```python
from build123d import *

# Parameters (mm, degrees)
SKETCH1_R                = 7
SKETCH1_R_2              = 3.5
CYLINDER_DEPTH           = 22.85
SKETCH2_R                = 4
BORE_1_DEPTH             = 3.25
BORE_START               = -3.25
SKETCH3_R                = 4
BORE_2_DEPTH             = 3.25
ARM_DEPTH                = 17
SKETCH5_R                = 3.5
OUTER_HOLE_SURFACE_DEPTH = 6
SKETCH6_R                = 1.125
OUTER_HOLE_DEPTH         = 6
SIDE_FEATURES_DEPTH      = 22
RIB_START                = -11
SKETCH10_W               = 6.681980515
SKETCH10_H               = 4.897943925
RIB_DEPTH                = 9.5
SKETCH13_R               = 1.5
BOTTOM_HOLE_DEPTH        = 4


# Read off the part's stored shape, not the designer's step: Top Counter-sunk
with BuildPart() as part:
    # Sketch1 → Cylinder (new body)
    with BuildSketch(Plane.XY):
        with Locations(Location((0, 0, 0), (0, 0, 180))):
            Circle(SKETCH1_R)
        with Locations(Location((0, 0, 0), (0, 0, 180))):
            Circle(SKETCH1_R_2, mode=Mode.SUBTRACT)
    extrude(amount=CYLINDER_DEPTH)

    # Sketch2 → Bore 1 (cut)
    with BuildSketch(Plane.XY.offset(22.85)):
        Circle(SKETCH2_R)
    extrude(amount=-BORE_1_DEPTH, mode=Mode.SUBTRACT)

    # Sketch3 → Bore 2 (cut)
    with BuildSketch(Plane(origin=(0, 0, 0), x_dir=(-1, 0, 0), z_dir=(0, 0, -1)).offset(BORE_START)):
        with Locations(Location((0, 0, 0), (0, 0, 180))):
            Circle(SKETCH3_R)
    extrude(amount=BORE_2_DEPTH, mode=Mode.SUBTRACT)

    # Sketch4 → Arm (add)
    with BuildSketch(Plane.XY):
        with BuildLine():
            Line((0.734153157, 6.961394914), (30, 3.875))
            ThreePointArc((30, 3.875), (33.875, 0), (30, -3.875))
            Line((30, -3.875), (0.734153157, -6.961394914))
            ThreePointArc((0.734153157, -6.961394914), (7, 0), (0.734153157, 6.961394914))
        make_face()
    extrude(amount=ARM_DEPTH)

    # Sketch5 → Outer Hole surface (add)
    with BuildSketch(Plane(origin=(0, 0, 0), x_dir=(-1, 0, 0), z_dir=(0, 0, -1))):
        with Locations((-14, 6)):
            Circle(SKETCH5_R)
    extrude(amount=-OUTER_HOLE_SURFACE_DEPTH)

    # Sketch6 → Outer hole (cut)
    with BuildSketch(Plane(origin=(0, 0, 0), x_dir=(-1, 0, 0), z_dir=(0, 0, -1))):
        with Locations((-14, 6)):
            Circle(SKETCH6_R)
    extrude(amount=-OUTER_HOLE_DEPTH, mode=Mode.SUBTRACT)

    # Sketch8 → side Features (cut)
    with BuildSketch(Plane(origin=(0, 10, 0), x_dir=(1, 0, 0), z_dir=(0, 1, 0))):
        with BuildLine():
            Line((21, -6), (40, -6))
            Line((40, -6), (40, -13))
            Line((40, -13), (21, -13))
            ThreePointArc((21, -13), (20.292893219, -12.707106781), (20, -12))
            Line((20, -12), (20, -7))
            ThreePointArc((20, -7), (20.292893219, -6.292893219), (21, -6))
        make_face()
        with BuildLine():
            Line((7, -19), (7, -9))
            Line((7, -9), (9.757359313, -9))
            ThreePointArc((9.757359313, -9), (10.90540961, -9.228361402), (11.878679656, -9.878679656))
            Line((11.878679656, -9.878679656), (17.535533906, -15.535533906))
            ThreePointArc((17.535533906, -15.535533906), (19.15765065, -16.619397663), (21.071067812, -17))
            Line((21.071067812, -17), (27, -17))
            Line((27, -17), (27, -19))
            Line((27, -19), (7, -19))
        make_face()
        Polygon((7, 0), (8.732050808, -1), (19, -1), (20.732050808, -2), (40, -2), (40, 0), align=None)
    extrude(amount=-SIDE_FEATURES_DEPTH, mode=Mode.SUBTRACT)

    # Sketch10 → Rib (cut)
    with BuildSketch(Plane.XY.offset(17).offset(RIB_START)):
        with Locations((14.159009743, 3.448971963)):
            Rectangle(SKETCH10_W, SKETCH10_H)
        with Locations((14.159009743, -3.448971963)):
            Rectangle(SKETCH10_W, SKETCH10_H)
    extrude(amount=RIB_DEPTH, mode=Mode.SUBTRACT)

    # Top Counter-sunk outline → Top Counter-sunk (revolve, cut)
    with BuildSketch(Plane(origin=(30, 0, 0), x_dir=(1, 0, 0), z_dir=(0, -1, 0))):
        Polygon((2, 3.150368407), (2, 6), (0, 6), (0, 2), (3, 2), align=None)
    revolve(axis=Axis((30, 0, 0), (0, 0, 1)), mode=Mode.SUBTRACT)

    # Sketch13 → Bottom hole (cut)
    with BuildSketch(Plane.XY.offset(17)):
        with Locations((30, 0)):
            Circle(SKETCH13_R)
    extrude(amount=-BOTTOM_HOLE_DEPTH, mode=Mode.SUBTRACT)


solid = part.part
```
Geometry check sheet. Reference: the model listing, model coordinates, mm. A direction names the side the tool comes from. Give positions to 0.01 mm unless a question says otherwise; leave off trailing zeros. Write each loop counter-clockwise with the first axis right and the second up, starting at its lowest first coordinate (ties: lowest second). Pieces come first, ordered by that corner, then holes. Notation, with made-up numbers: (29.5, 86.25) -> (62.5, 86.25) arc R24 cw to (62.5, 118.25) -> close; hole circle Ø4 at (47.25, 18.25). An arc over 180 degrees is marked (long way). Use one line per item in the form item = value.
Item 1: Sectioned sample at A-A on x = 0. Enter the section's corners in (y, z).
Results list:
outline = (-7, 0) -> (-4, 0) -> (-4, 3.25) -> (-3.5, 3.25) -> (-3.5, 19.6) -> (-4, 19.6) -> (-4, 22.85) -> (-7, 22.85) -> close; (3.5, 3.25) -> (4, 3.25) -> (4, 0) -> (7, 0) -> (7, 22.85) -> (4, 22.85) -> (4, 19.6) -> (3.5, 19.6) -> close
Item 2: Sectioned sample at C-C on x = 14. Enter the section's corners in (y, z) (3 decimals), plus the area to 3 significant figures.
Results list:
outline = (-5.562, 1) -> (4.875, 1) -> (4.875, 6) -> (1, 6) -> (1, 12) -> (-1, 12) -> (-1, 6) -> (-5.562, 6) -> close; (7.125, 1) -> (9.5, 1) -> (9.5, 6) -> (7.125, 6) -> close
area = 76.1 mm2
Item 3: Access from +Z, -Z, +X, -X, +Y, -Y to the whole of each face (thin tool, end or side, straight path). Record for faces 1 (the cylindrical face through (20.285, 0.069, 6.301)), 2 (the cylindrical face through (19.13, 0.07, 16.61)), 3 (the cylindrical face through (-6.677, -2.103, 13.804)), 4 (the flat face through (17.5, 3, 11)).
Results list:
face_1 = +X, +Y, -Y
face_2 = +Z, +Y, -Y
face_3 = +Z
face_4 = +Z, +Y
Item 4: Sectioned sample at D-D on y = 8.5. Enter the section's corners in (x, z), plus the area to 3 significant figures.
Results list:
outline = (11.55, 1) -> (16.45, 1) -> (16.45, 6) -> (11.55, 6) -> close
area = 24.5 mm2
Item 5: Scan lines: line 1 (Y direction, x = 0, z = 2); line 2 (Z direction, x = 14, y = 1.5); line 3 (X direction, y = -2.5, z = 7). Record each from-to range of solid material in increasing order.
Results list:
line_1 = -7 to -4, 4 to 7
line_2 = 1 to 6
line_3 = -6.54 to -2.45, 2.45 to 10.82, 17.5 to 20
Item 6: Mould release check, pull along Y, two halves, no side actions. Record for faces 5 (the flat face through (20, 0, 10)), 6 (the cylindrical face through (33.874, 0.085, 3.972)), 7 (the cylindrical face through (-0.867, 3.905, 1.648)), 8 (the flat face through (15, -1, 10)): released by +Y, released by -Y, zero draft, split by the parting line, or undercut.
Results list:
face_5 = zero draft
face_6 = split by the parting line
face_7 = undercut
face_8 = released by -Y
Item 7: Depth check by flat-ended pin: pin 1 Ø3 at (x, y) = (29, -2) entering from -Z; pin 2 Ø6 at (x, y) = (19, -4) entering from -Z; pin 3 Ø1.4 at (x, y) = (8.5, 0) entering from +Z. Enter the tip coordinate at first touch or a pass-through.
Results list:
pin_1 = 2
pin_2 = 1
pin_3 = 9
Item 8: Sectioned sample at B-B on z = 21. Enter the section's corners in (x, y), plus the area to 3 significant figures.
Results list:
outline = circle Ø14 at (0, 0); hole circle Ø8 at (0, 0)
area = 104 mm2
